Read the model definition and answer for the solid it produces. Units are mm, in the model's axes. A direction names the side the tool comes from. Round coordinates to 2 decimals unless told otherwise and drop trailing zeros. Write each loop counter-clockwise with the first axis right and the second up, starting at its lowest first coordinate (ties: lowest second). Pieces come first, ordered by that corner, then holes. Notation, with made-up numbers: (11, 39.25) -> (54, 39.25) arc R24 ccw to (54, 67.25) -> close; hole circle Ø6 at (5.25, 82.5). An arc over 180 degrees is marked (long way). Return JSON: item names as keys, results as strings. Group by question number.
(1) A cutting plane is placed at B-B on y = -8.5. Give the vertices of the cut face in (x, z).
(2) Given pin 1 (8 mm diameter, centred on x = 64, y = -7.5, fed in from -Z); pin 2 (21 mm diameter, centred on x = 39.5, y = -10.5, fed in from +Z), each flat-ended and moving along its own axis, determine where each tip first touches the part or whether it passes through.
(3) A cutting plane is placed at A-A on x = -63. Give the vertices of the cut face in (y, z), then the cut area to 3 significant figures.
(4) Straight lines are drawn through the part: line 1 (X direction, y = -14, z = 10.5); line 2 (Y direction, x = -10.5, z = 12.25); line 3 (X direction, y = 15, z = 2.5). For each, find the intervals that lie inside material, in ascending order.
(5) For faces 4 (the flat face through (-123.5, 0, 6)), 5 (the flat face through (-2, 21.25, 8)), determine the directions among +Z, -Z, +X, -X, +Y, -Y from which every point of the face is accessible in a straight line to the end or side of a thin tool.
(6) A cutting plane is placed at C-C on z = 8. Give the vertices of the cut face in (x, y), then the cut area to 3 significant figures.
(7) The mould has two halves that part along Y. Classify faces 1 (the flat face through (113.5, 0, 8)), 2 (the flat face through (-2, -29, 6)), 3 (the flat face through (-2, -19, 0)): released by +Y, released by -Y, zero draft, split by the parting line, or undercut.
```python
from build123d import *

# Parameters (mm, degrees)
F0_W     = 227
F0_H     = 42.5
F0_W_2   = 142
F0_H_2   = 35.5
F1_DEPTH = 3
F0_W_3   = 247
F0_H_3   = 58
F2_DEPTH = 13
F3_SIZE  = 0.5
F4_SIZE  = 0.5


with BuildPart() as f1:
    # F0 (on Top) → F1 (new body)
    with BuildSketch(Plane.XY):
        Rectangle(F0_W, F0_H)
        Rectangle(F0_W_2, F0_H_2, mode=Mode.SUBTRACT)
    extrude(amount=F1_DEPTH)

    # F0 (on Top) → F2 (join)
    with BuildSketch(Plane.XY):
        Rectangle(F0_W_3, F0_H_3)
        Rectangle(F0_W, F0_H, mode=Mode.SUBTRACT)
    extrude(amount=F2_DEPTH)

    # F3
    f3_edges = [f1.edges().sort_by_distance(p)[0] for p in [
        (-123.5, -29, 6.5),
        (0, -29, 13),
        (123.5, 0, 13),
        (0, 29, 13),
        (-123.5, 0, 13),
        (113.5, 0, 13),
        (0, -21.25, 13),
        (-113.5, 0, 13),
        (0, 21.25, 13),
        (123.5, -29, 6.5),
        (123.5, 29, 6.5),
        (-123.5, 29, 6.5),
        (-123.5, 0, 0),
        (0, -29, 0),
        (0, 29, 0),
        (123.5, 0, 0),
    ]]
    chamfer(f3_edges, length=F3_SIZE)

    # F4
    f4_edges = [f1.edges().sort_by_distance(p)[0] for p in [
        (0, -17.75, 3),
        (-71, 0, 3),
        (0, 17.75, 3),
        (71, 0, 3),
        (0, -17.75, 0),
        (-71, 0, 0),
        (0, 17.75, 0),
        (71, 0, 0),
    ]]
    chamfer(f4_edges, length=F4_SIZE)


solid = f1.part
```
Checks:
{
 "1": {"outline": "(-123.5, 0.5) -> (-123, 0) -> (-71.5, 0) -> (-71, 0.5) -> (-71, 2.5) -> (-71.5, 3) -> (-113.5, 3) -> (-113.5, 12.5) -> (-114, 13) -> (-123, 13) -> (-123.5, 12.5) -> close; (71, 0.5) -> (71.5, 0) -> (123, 0) -> (123.5, 0.5) -> (123.5, 12.5) -> (123, 13) -> (114, 13) -> (113.5, 12.5) -> (113.5, 3) -> (71.5, 3) -> (71, 2.5) -> close"},
 "2": {"pin 1": "passes through", "pin 2": "stops at z = 3"},
 "3": {"outline": "(-29, 0.5) -> (-28.5, 0) -> (-18.25, 0) -> (-17.75, 0.5) -> (-17.75, 2.5) -> (-18.25, 3) -> (-21.25, 3) -> (-21.25, 12.5) -> (-21.75, 13) -> (-28.5, 13) -> (-29, 12.5) -> close; (17.75, 0.5) -> (18.25, 0) -> (28.5, 0) -> (29, 0.5) -> (29, 12.5) -> (28.5, 13) -> (21.75, 13) -> (21.25, 12.5) -> (21.25, 3) -> (18.25, 3) -> (17.75, 2.5) -> close", "area": "221 mm^2"},
 "4": {"line 1": "x = -123.5 to -113.5, 113.5 to 123.5", "line 2": "y = -29 to -21.25, 21.25 to 29", "line 3": "x = -123.5 to -71, 71 to 123.5"},
 "5": {"face 4": "+Z, -Z, -X, +Y, -Y", "face 5": "+Z"},
 "6": {"outline": "(-123.5, -28.5) -> (-123, -29) -> (123, -29) -> (123.5, -28.5) -> (123.5, 28.5) -> (123, 29) -> (-123, 29) -> (-123.5, 28.5) -> close; hole (-113.5, -21.25) -> (113.5, -21.25) -> (113.5, 21.25) -> (-113.5, 21.25) -> close", "area": "4,680 mm^2"},
 "7": {"face 1": "undercut", "face 2": "released by -Y", "face 3": "zero draft"}
}
